from build123d import *

# Parameters (mm, degrees)
F1_DEPTH = 12.7
F2_W     = 3
F2_H     = 27
F2_W_2   = 7.2
F2_H_2   = 20
F3_DEPTH = 1
F4_R     = 3


with BuildPart() as f1:
    # F0 (on Right) → F1 (new body, symmetric)
    with BuildSketch(Plane.YZ):
        Polygon((6.7, 0), (0, 0), (0, -27), (1, -27), (1, -1), (5.7, -1), (5.7, -3.5), (6.7, -3.5), align=None)
    extrude(amount=F1_DEPTH, both=True)

    # F2 (on face) → F3 (cut, through all)
    with BuildSketch(Plane.XZ):
        with Locations((0, -13.5)):
            Rectangle(F2_W, F2_H)
        with Locations((-9.1, -17)):
            Rectangle(F2_W_2, F2_H_2)
        with Locations((9.1, -17)):
            Rectangle(F2_W_2, F2_H_2)
    extrude(amount=-F3_DEPTH, mode=Mode.SUBTRACT)

    # F4
    f4_edges = [f1.edges().sort_by_distance(p)[0] for p in [
        (5.5, 0.5, -27),
        (-5.5, 0.5, -27),
        (-5.5, 0.5, -7),
        (-12.7, 0.5, -7),
        (5.5, 0.5, -7),
        (12.7, 0.5, -7),
    ]]
    fillet(f4_edges, radius=F4_R)


solid = f1.part
Geometry check sheet. Reference: the model listing, model coordinates, mm. A direction names the side the tool comes from. Round coordinates to 2 decimals unless told otherwise and drop trailing zeros. Order: outer loops, then holes, each group sorted by start corner. A loop starts at its lowest first (then second) coordinate and runs counter-clockwise, first axis right, second up. Notation, with made-up numbers: M 71,69 L 115,69 A17 cw 115,80 Z; hole C -34,-9 d6. An arc over 180 degrees is marked long. Answer in a Markdown table with one row per item. Add a question column.
Item 1: Set-up check for faces 5 (the face through (0, 3, -1)), 6 (the face through (-9.1, 0.5, -7)), 7 (the face through (5.5, 0.5, -17.1)): record each of +Z, -Z, +X, -X, +Y, -Y from which the full face is reachable in a straight line by a thin tool's end or side.
Item 2: Sectioned sample at B-B, the plane x = 9. Enter the section's corners in (y, z), plus the area to 3 significant figures.
Item 3: Draft check along X on faces 1 (the face through (-4.6, 0.51, -26.14)), 2 (the face through (0, 1, -0.5)), 3 (the face through (0, 6, -3.5)), 4 (the face through (11.84, 0.51, -6.1)). Enter one of: released by +X, released by -X, zero draft, split by the parting line, or undercut.
Item 4: Depth check by flat-ended pin: pin 1 Ø9 at (x, z) = (-8.5, -8.5) entering from +Y; pin 2 Ø4 at (x, y) = (1, 6) entering from +Z; pin 3 Ø0.8 at (y, z) = (0.5, -16) entering from +X; pin 4 Ø0.8 at (x, y) = (9, 0.5) entering from -Z. Enter the tip coordinate at first touch or a pass-through.
Item 5: Material ranges on L1, parallel to X at y = 0.5, z = -11.5; L2, parallel to Y at x = 2.5, z = -1.75; L3, parallel to Z at x = 3.75, y = 4.5, recorded low to high. Write a range as [from, to].
Item 6: Sectioned sample at D-D, the plane y = 4.5. Enter the section's corners in (x, z), plus the area to 3 significant figures.
Item 7: Sectioned sample at A-A, the plane z = -19. Enter the section's corners in (x, y).
Item 8: Sectioned sample at C-C, the plane z = -9. Enter the section's corners in (x, y).
Filled in:
| question | item | result |
|---|---|---|
| 1 | face 5 | -Z, +X, -X |
| 1 | face 6 | -Z, -X, +Y, -Y |
| 1 | face 7 | -Z, +X, +Y, -Y |
| 2 | outline | M 0,-7 L 1,-7 L 1,-1 L 5.7,-1 L 5.7,-3.5 L 6.7,-3.5 L 6.7,0 L 0,0 Z |
| 2 | area | 15.2 mm² |
| 3 | face 1 | released by -X |
| 3 | face 2 | undercut |
| 3 | face 3 | zero draft |
| 3 | face 4 | released by +X |
| 4 | pin 1 | stops at y = 1 |
| 4 | pin 2 | stops at z = 0 |
| 4 | pin 3 | stops at x = 5.5 |
| 4 | pin 4 | stops at z = -7 |
| 5 | L1 | x = [-5.5, -1.5], [1.5, 5.5] |
| 5 | L2 | y = [0, 1], [5.7, 6.7] |
| 5 | L3 | z = [-1, 0] |
| 6 | outline | M -12.7,-1 L 12.7,-1 L 12.7,0 L -12.7,0 Z |
| 6 | area | 25.4 mm² |
| 7 | outline | M -5.5,0 L -1.5,0 L -1.5,1 L -5.5,1 Z; M 1.5,0 L 5.5,0 L 5.5,1 L 1.5,1 Z |
| 8 | outline | M -5.67,0 L -1.5,0 L -1.5,1 L -5.67,1 Z; M 1.5,0 L 5.67,0 L 5.67,1 L 1.5,1 Z |
